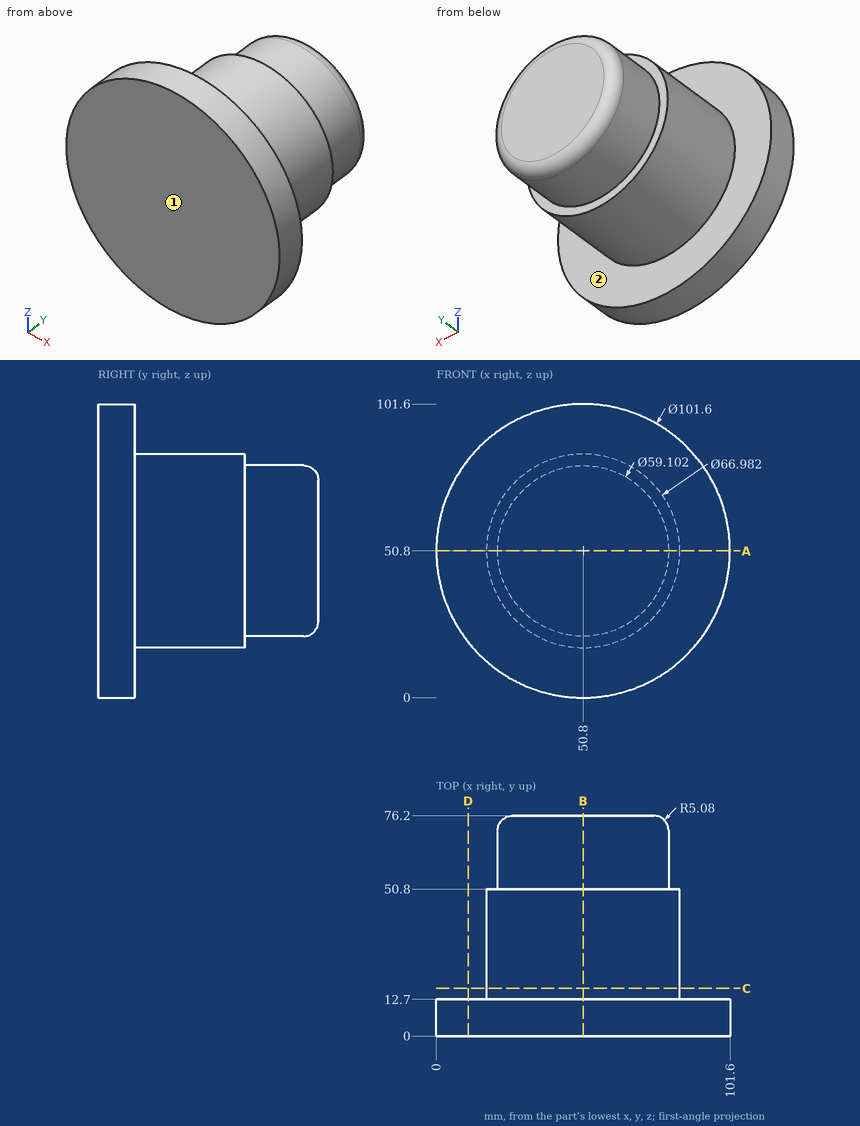
Geometry check sheet. Reference: drawing and pictorial views, mm from the part's lowest x, y, z. A direction names the side the tool comes from. Give positions to 0.01 mm unless a question says otherwise; leave off trailing zeros. Write each loop counter-clockwise with the first axis right and the second up, starting at its lowest first coordinate (ties: lowest second). Pieces come first, ordered by that corner, then holes. Notation, with made-up numbers: (10, 70.5) - (31, 70.5) arc R33 cw to (31, 108.5) - close; hole circle Ø10 at (53.25, 87). An arc over 180 degrees is marked (long way). Use a Markdown table: item, result.
Q1. Go/stop test with flat-tipped pins: P1, Ø3, axis at x = 66.5, y = 53.5, coming from the -Z side (1 decimal); P2, Ø10, axis at x = 46, y = 9, coming from the +Z side; P3, Ø1.5, axis at x = 40.5, z = 74, coming from the +Y side. Record where each tip stops, or that it passes through.
Computed:
| item | result |
|---|---|
| P1 | stops at z = 24.9 |
| P2 | stops at z = 101.6 |
| P3 | stops at y = 76.2 |
Q2. Section check C-C, the plane y = 16.5. Enter the section's corners in (x, z), then the cut area to 3 significant figures.
Computed:
| item | result |
|---|---|
| outline | circle Ø66.98 at (50.8, 50.8) |
| area | 3,520 mm² |
Q3. Section check B-B, the plane x = 50.8. Enter the section's corners in (y, z).
Computed:
| item | result |
|---|---|
| outline | (0, 0) - (12.7, 0) - (12.7, 17.31) - (50.8, 17.31) - (50.8, 21.25) - (71.12, 21.25) arc R5.08 ccw to (76.2, 26.33) - (76.2, 75.27) arc R5.08 ccw to (71.12, 80.35) - (50.8, 80.35) - (50.8, 84.29) - (12.7, 84.29) - (12.7, 101.6) - (0, 101.6) - close |
Q4. Set-up check for the marked faces 1 and 2: record each of +Z, -Z, +X, -X, +Y, -Y from which the full face is reachable in a straight line by a thin tool's end or side.
Computed:
| item | result |
|---|---|
| face 1 | +Z, -Z, +X, -X, -Y |
| face 2 | +Y |
Q5. Section check A-A, the plane z = 50.8. Enter the section's corners in (x, y).
Computed:
| item | result |
|---|---|
| outline | (0, 0) - (101.6, 0) - (101.6, 12.7) - (84.29, 12.7) - (84.29, 50.8) - (80.35, 50.8) - (80.35, 71.12) arc R5.08 ccw to (75.27, 76.2) - (26.33, 76.2) arc R5.08 ccw to (21.25, 71.12) - (21.25, 50.8) - (17.31, 50.8) - (17.31, 12.7) - (0, 12.7) - close |
Q6. Thickness scan on L1, parallel to Y at x = 7, z = 45; L2, parallel to Y at x = 36.5, z = 22; L3, parallel to X at y = 26, z = 28. Record the ranges inside material, lowest first. Write a range as [from, to].
Computed:
| item | result |
|---|---|
| L1 | y = [0, 12.7] |
| L2 | y = [0, 50.8] |
| L3 | x = [26.27, 75.33] |
Q7. Section check D-D, the plane x = 11. Enter the section's corners in (y, z).
Computed:
| item | result |
|---|---|
| outline | (0, 19.23) - (12.7, 19.23) - (12.7, 82.37) - (0, 82.37) - close |
